Drawing for the job (mm, zero at the part's lowest x, y, z). A direction names the side the tool comes from. Round coordinates to 2 decimals unless told otherwise and drop trailing zeros. Write each loop counter-clockwise with the first axis right and the second up, starting at its lowest first coordinate (ties: lowest second). Pieces come first, ordered by that corner, then holes.
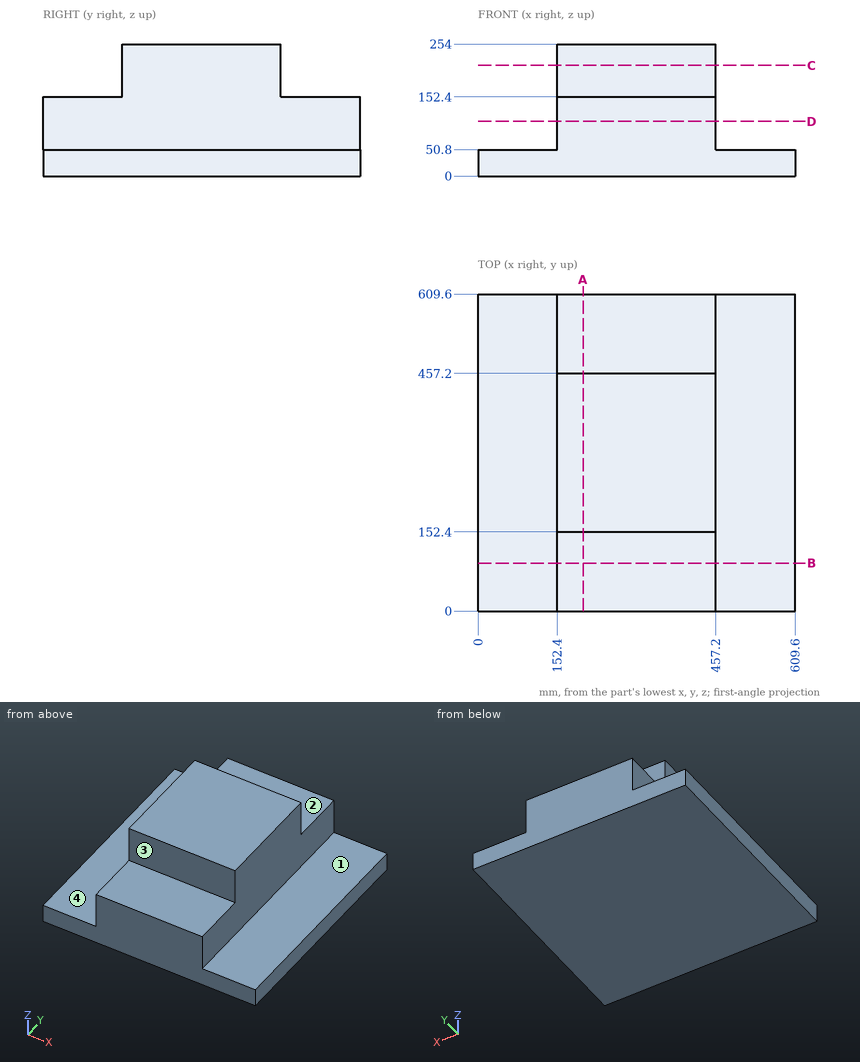
Q1. Saw through at A-A, the plane x = 202. Write the cut outline in (y, z).
Q2. Saw through at C-C, the plane z = 213. Write the cut outline in (x, y).
Q3. Saw through at D-D, the plane z = 105. Write the cut outline in (x, y), and give its area (3 significant figures).
Q4. Drop flat-ended pins along their axis: P1, Ø8, axis at x = 429, y = 459.5, coming from the +Z side; P2, Ø4, axis at y = 242.5, z = 139, coming from the -X side. Give the stop position or say it passes through.
Q5. Wall check: line 1 (Y direction, x = 398, z = 189); line 2 (Z direction, x = 97, y = 365). Give the ranges that are in metal, low to high.
Q6. Saw through at B-B, the plane y = 92. Write the cut outline in (x, z), and give its area (3 significant figures).
Q7. Tool access for the marked faces 1, 2, 3 and 4: list every direction of +Z, -Z, +X, -X, +Y, -Y with a clear straight run to the whole face (end or side of a thin tool).
Computed:
1. outline: (0, 0) - (609.6, 0) - (609.6, 152.4) - (457.2, 152.4) - (457.2, 254) - (152.4, 254) - (152.4, 152.4) - (0, 152.4) - close
2. outline: (152.4, 152.4) - (457.2, 152.4) - (457.2, 457.2) - (152.4, 457.2) - close
3. outline: (152.4, 0) - (457.2, 0) - (457.2, 609.6) - (152.4, 609.6) - close
3. area: 186,000 mm2
4. P1: stops at z = 254
4. P2: stops at x = 152.4
5. line 1: y = 152.4 to 457.2
5. line 2: z = 0 to 50.8
6. outline: (0, 0) - (609.6, 0) - (609.6, 50.8) - (457.2, 50.8) - (457.2, 152.4) - (152.4, 152.4) - (152.4, 50.8) - (0, 50.8) - close
6. area: 61,900 mm2
7. face 1: +Z, +X, +Y, -Y
7. face 2: +Z, +X, -X, +Y
7. face 3: +Z, +X, -X, -Y
7. face 4: +Z, -X, +Y, -Y
